Read the model definition and answer for the solid it produces. Units are mm, in the model's axes. Coordinates: 2 decimals unless noted, no trailing zeros. Loops run counter-clockwise (first coordinate to the right, second up) from the corner with the lowest first, then second, coordinate; pieces in that order, holes last. Notation, with made-up numbers: (46.5, -24.75) -> (81.5, -24.75) arc R13 ccw to (81.5, -20.75) -> close; hole circle Ø7 at (21.25, 76). An arc over 180 degrees is marked (long way). Answer as a JSON object with one key per item and string values. Group by question number.
1) A flat-ended cylindrical pin translates along its axis: P1, Ø4, axis at y = 451, z = 11.5, coming from the -X side. Find the tip coordinate at first contact, or state that the pin passes through.
2) Section C-C, the plane x = 494 is taken. Give the vertices of the cut face in (y, z), plus the area to 3 significant figures.
3) Section A-A, the plane z = 5.5 is taken. Give the vertices of the cut face in (x, y).
4) Section B-B, the plane y = 383 is taken. Give the vertices of the cut face in (x, z), plus the area to 3 significant figures.
5) Consider probe 1 along X at (y, z) = (357.5, 8.25); probe 2 along Y at (x, z) = (202, 11.5); probe 3 along X at (y, z) = (147, 10.75). Determine where each line is inside the solid, lowest interval first. Write a range as [from, to].
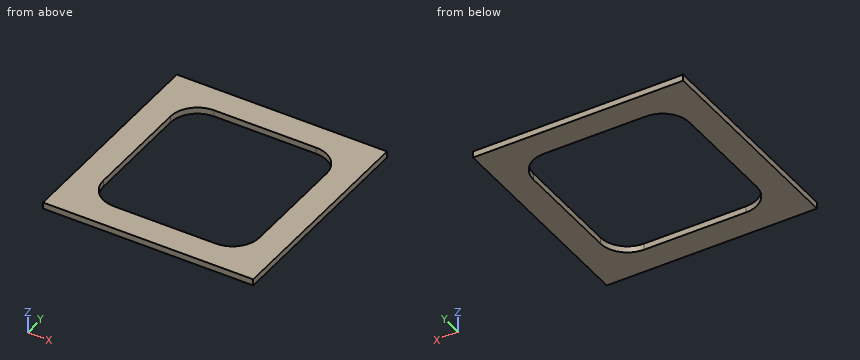
from build123d import *

# Parameters (mm, degrees)
F0_W     = 592.3788
F0_H     = 609.6
F1_DEPTH = 18.034
F2_W     = 439.9788
F2_H     = 457.2
F3_DEPTH = 18.035
F4_R     = 76.2


with BuildPart() as f1:
    # F0 (on Top) → F1 (new body)
    with BuildSketch(Plane.XY):
        with Locations((296.1894, 304.8)):
            Rectangle(F0_W, F0_H)
    extrude(amount=F1_DEPTH)

    # F2 (on face) → F3 (cut, through all)
    with BuildSketch(Plane.XY.offset(18.034)):
        with Locations((296.1894, 304.8)):
            Rectangle(F2_W, F2_H)
    extrude(amount=-F3_DEPTH, mode=Mode.SUBTRACT)

    # F4
    f4_edges = [f1.edges().sort_by_distance(p)[0] for p in [
        (516.1788, 533.4, 9.017),
        (76.2, 533.4, 9.017),
        (76.2, 76.2, 9.017),
        (516.1788, 76.2, 9.017),
    ]]
    fillet(f4_edges, radius=F4_R)


solid = f1.part
Determined:
{
 "1": {"P1": "x = 0"},
 "2": {"outline": "(0, 0) -> (98.66, 0) -> (98.66, 18.03) -> (0, 18.03) -> close; (510.94, 0) -> (609.6, 0) -> (609.6, 18.03) -> (510.94, 18.03) -> close", "area": "3,560 mm²"},
 "3": {"outline": "(0, 0) -> (592.38, 0) -> (592.38, 609.6) -> (0, 609.6) -> close; hole (76.2, 152.4) arc R76.2 ccw to (152.4, 76.2) -> (439.98, 76.2) arc R76.2 ccw to (516.18, 152.4) -> (516.18, 457.2) arc R76.2 ccw to (439.98, 533.4) -> (152.4, 533.4) arc R76.2 ccw to (76.2, 457.2) -> close"},
 "4": {"outline": "(0, 0) -> (76.2, 0) -> (76.2, 18.03) -> (0, 18.03) -> close; (516.18, 0) -> (592.38, 0) -> (592.38, 18.03) -> (516.18, 18.03) -> close", "area": "2,750 mm²"},
 "5": {"probe 1": "[0, 76.2], [516.18, 592.38]", "probe 2": "[0, 76.2], [533.4, 609.6]", "probe 3": "[0, 76.39], [515.99, 592.38]"}
}
